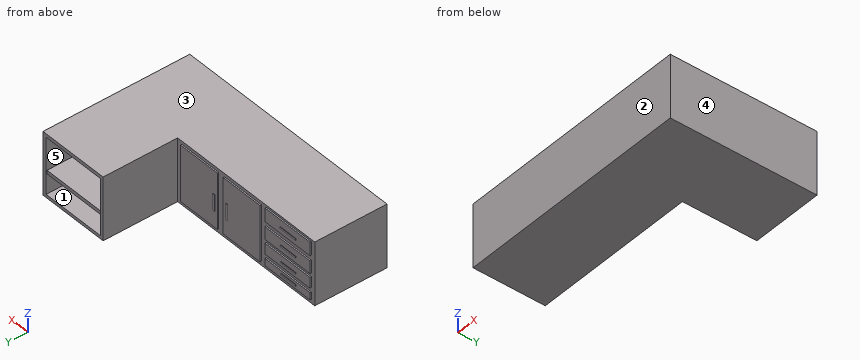
from build123d import *

# Parameters (mm, degrees)
F1_DEPTH = 426.72
F2_W     = 365.76
F2_H     = 48.768
F2_H_2   = 73.152
F2_H_3   = 85.344
F2_H_4   = 91.44
F2_W_2   = 298.704
F2_H_5   = 377.952
F3_DEPTH = 9.144
F4_W     = 119.230599
F4_H     = 11.923056
F4_H_2   = 9.935886
F4_W_2   = 123.204947
F4_H_3   = 11.92306
F4_W_3   = 127.179295
F4_H_4   = 11.923045
F4_W_4   = 15.897393
F4_H_5   = 109.294712
F4_W_5   = 17.884612
F5_DEPTH = 12.192
F6_W     = 439.548612
F6_H     = 382.832659
F7_DEPTH = 359.664
F8_W     = 439.548612
F8_H     = 23.631648
F9_DEPTH = 353.568


with BuildPart() as f1:
    # F0 (on Top) → F1 (new body)
    with BuildSketch(Plane.XY):
        Polygon((0, 487.68), (0, 0), (1600.2, 0), (1600.2, 990.6), (1112.52, 990.6), (1112.52, 487.68), align=None)
    extrude(amount=F1_DEPTH)

    # F2 (on face) → F3 (join)
    with BuildSketch(Plane(origin=(0, 487.68, 0), x_dir=(-1, 0, 0), z_dir=(0, 1, 0))):
        with Locations((-210.133546, 51.409847)):
            Rectangle(F2_W, F2_H)
        with Locations((-210.133546, 141.325856)):
            Rectangle(F2_W, F2_H_2)
        with Locations((-210.133546, 245.719852)):
            Rectangle(F2_W, F2_H_3)
        with Locations((-210.133546, 367.639854)):
            Rectangle(F2_W, F2_H_4)
        with Locations((-582.587673, 216.001847)):
            Rectangle(F2_W_2, F2_H_5)
        with Locations((-928.356364, 216.001847)):
            Rectangle(F2_W_2, F2_H_5)
    extrude(amount=F3_DEPTH)

    # F4 (on face) → F5 (join)
    with BuildSketch(Plane(origin=(0, 487.68, 0), x_dir=(-1, 0, 0), z_dir=(0, 1, 0))):
        with Locations((-202.043369, 52.071078)):
            Rectangle(F4_W, F4_H)
        with Locations((-202.043369, 132.55173)):
            Rectangle(F4_W, F4_H_2)
        with Locations((-204.030543, 240.852855)):
            Rectangle(F4_W_2, F4_H_3)
        with Locations((-206.017718, 360.083445)):
            Rectangle(F4_W_3, F4_H_4)
        with Locations((-702.811837, 192.167029)):
            Rectangle(F4_W_4, F4_H_5)
        with Locations((-807.138622, 192.167029)):
            Rectangle(F4_W_5, F4_H_5)
    extrude(amount=F5_DEPTH)

    # F6 (on face) → F7 (cut)
    with BuildSketch(Plane(origin=(0, 990.6, 0), x_dir=(-1, 0, 0), z_dir=(0, 1, 0))):
        with Locations((-1355.178416, 212.191843)):
            Rectangle(F6_W, F6_H)
    extrude(amount=-F7_DEPTH, mode=Mode.SUBTRACT)

    # F8 (on face) → F9 (join)
    with BuildSketch(Plane(origin=(0, 630.936, 0), x_dir=(-1, 0, 0), z_dir=(0, 1, 0))):
        with Locations((-1355.178416, 167.291738)):
            Rectangle(F8_W, F8_H)
    extrude(amount=F9_DEPTH)


solid = f1.part
Source: CAD feature listing. Evaluate the final solid. Frame: model axes, mm. Face numbers are marked on the shaded views. A direction names the side the tool comes from. Coordinates: 2 decimals unless noted, no trailing zeros. Order: outer loops, then holes, each group sorted by start corner. A loop starts at its lowest first (then second) coordinate and runs counter-clockwise, first axis right, second up. Notation, with made-up numbers: M -7,79 L 14,79 A18 cw 14,85 Z; hole C 75,37 d3. An arc over 180 degrees is marked long. Write each question's results on one line, items separated by ' | '. Start each with the question number.
1. Section D-D, the plane x = 1258. Return the cut outline in (y, z).
2. Reachability of the marked faces 1 and 2 from +Z, -Z, +X, -X, +Y, -Y: full face, straight path, thin tool, end or side. Return the list, or none.
3. Draft query along Z for the marked faces 3, 4 and 5. Return one class per face: +Z half, -Z half, draft (parallel to the pull), parting line (faces both ways), or undercut.
4. Section A-A, the plane x = 996. Return the cut outline in (y, z).
5. Section C-C, the plane x = 288. Return the cut outline in (y, z).
6. Material intervals for L1, parallel to X at y = 825, z = 28; L2, parallel to X at y = 607, z = 134.5; L3, parallel to Y at x = 217, z = 369, sorted ascending.
7. Pin query (flat end, axial travel): pin 1 (2.5 mm diameter, centred on x = 915.5, y = 494.5, fed in from -Z); pin 2 (1.5 mm diameter, centred on y = 497.5, z = 131.5, fed in from -X); pin 3 (4 mm diameter, centred on x = 419, z = 279.5, fed in from +Y). Return the tip coordinate at first contact, or that it passes through.
8. Section B-B, the plane y = 836. Return the cut outline in (x, z), then the cut area to 3 significant figures.
Solution:
1) outline: M 0,0 L 990.6,0 L 990.6,20.78 L 630.94,20.78 L 630.94,155.48 L 984.5,155.48 L 984.5,179.11 L 630.94,179.11 L 630.94,403.61 L 990.6,403.61 L 990.6,426.72 L 0,426.72 Z
2) face 1: +Y | face 2: +Z, -Z, +X, -X, -Y
3) face 3: +Z half | face 4: draft | face 5: undercut
4) outline: M 0,0 L 487.68,0 L 487.68,27.03 L 496.82,27.03 L 496.82,404.98 L 487.68,404.98 L 487.68,426.72 L 0,426.72 Z
5) outline: M 0,0 L 487.68,0 L 487.68,27.03 L 496.82,27.03 L 496.82,75.79 L 487.68,75.79 L 487.68,104.75 L 496.82,104.75 L 496.82,177.9 L 487.68,177.9 L 487.68,203.05 L 496.82,203.05 L 496.82,288.39 L 487.68,288.39 L 487.68,321.92 L 496.82,321.92 L 496.82,413.36 L 487.68,413.36 L 487.68,426.72 L 0,426.72 Z
6) L1: 1112.52 to 1135.4, 1574.95 to 1600.2 | L2: 1112.52 to 1600.2 | L3: 0 to 496.82
7) pin 1: z = 27.03 | pin 2: x = 27.25 | pin 3: y = 487.68
8) outline: M 1112.52,0 L 1600.2,0 L 1600.2,426.72 L 1112.52,426.72 Z; hole M 1135.4,20.78 L 1574.95,20.78 L 1574.95,155.48 L 1135.4,155.48 Z; hole M 1135.4,179.11 L 1574.95,179.11 L 1574.95,403.61 L 1135.4,403.61 Z | area: 50,200 mm²
